Geometry: final body of the model. Coordinates: model frame, mm. Face numbers are marked on the shaded views. A direction names the side the tool comes from. Coordinates: 2 decimals unless noted, no trailing zeros. Order: outer loops, then holes, each group sorted by start corner. A loop starts at its lowest first (then second) coordinate and runs counter-clockwise, first axis right, second up. Notation, with made-up numbers: M 79,12 L 113,12 A22 ccw 113,40 Z; hole C 12,-7 d8. An arc over 180 degrees is marked long. Use CSV: the item, a comma, the result in double quotes. Start each with the question number.
1. Section query C-C on x = -75. Return the cut outline in (y, z).
2. Material intervals for line 1 (Z direction, x = 47, y = 3.25); line 2 (Y direction, x = -106.8, z = 52.5); line 3 (X direction, y = 7.75, z = 43), sorted ascending.
3. Section query A-A on x = 53. Return the cut outline in (y, z), and give its area (3 significant figures).
4. Section query B-B on z = 22.5. Return the cut outline in (x, y).
5. First-contact query: P1, Ø3, axis at x = -66.51, z = 0.57, coming from the -Y side; P2, Ø4, axis at x = 62, z = 74.5, coming from the +Y side; P3, Ø4.5, axis at x = 75, y = 5, coming from the +Z side; P4, Ø3.5, axis at x = 75, y = 5, coming from the -Z side. Flat tips, straight axial feed; report the tip coordinate or a pass-through.
6. Set-up query: the marked faces 1 and 2. Return all of +Z, -Z, +X, -X, +Y, -Y with unobstructed straight access to the full face (end or side cutting, diameter ignored); none if empty.
7. Section query D-D on z = 43. Return the cut outline in (x, y), and give its area (3 significant figures).
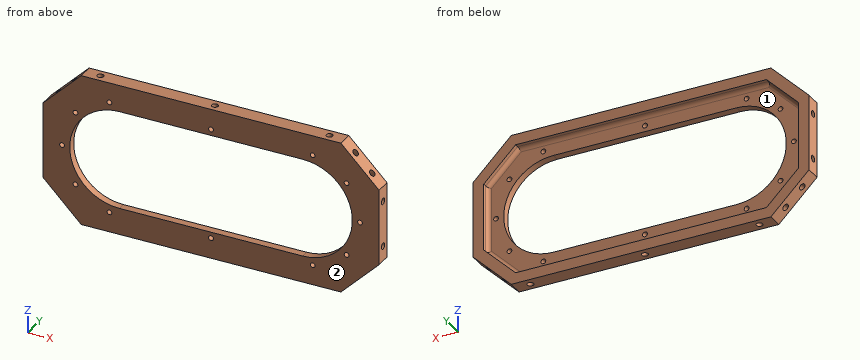
from build123d import *

# Parameters (mm, degrees)
MAIN_DEPTH                                     = 10
SKETCH3_R                                      = 1.55
ACTUATOR_SCREW_HOLE_DEPTH                      = 141.91220671
ACTUATOR_SCREW_HOLE_PATTERN_COUNT              = 3
ACTUATOR_SCREW_HOLE_PATTERN_ANGLE              = 80
ACTUATOR_SCREW_HOLE_PATTERN_THE_OTHER_WA_COUNT = 3
ACTUATOR_SCREW_HOLE_PATTERN_THE_OTHER_WA_ANGLE = 80
DISH_DEPTH                                     = 5
DISH_FILLET_R                                  = 2.5
F_4_0MM_DOWEL_HOLE1_D                          = 4.1
F_4_0MM_DOWEL_HOLE1_DEPTH                      = 5.7
F_4_0MM_DOWEL_HOLE1_ON_FACE_2_D                = 4.1
F_4_0MM_DOWEL_HOLE1_ON_FACE_2_DEPTH            = 5.7
F_4_0MM_DOWEL_HOLE1_ON_FACE_3_D                = 4.1
F_4_0MM_DOWEL_HOLE1_ON_FACE_3_DEPTH            = 5.7
F_4_0MM_DOWEL_HOLE1_ON_FACE_4_D                = 4.1
F_4_0MM_DOWEL_HOLE1_ON_FACE_4_DEPTH            = 5.7
F_4_0MM_DOWEL_HOLE1_ON_FACE_5_D                = 4.1
F_4_0MM_DOWEL_HOLE1_ON_FACE_5_DEPTH            = 5.7
F_4_0MM_DOWEL_HOLE1_ON_FACE_6_D                = 4.1
F_4_0MM_DOWEL_HOLE1_ON_FACE_6_DEPTH            = 5.7
F_4_0MM_DOWEL_HOLE1_ON_FACE_7_D                = 4.1
F_4_0MM_DOWEL_HOLE1_ON_FACE_7_DEPTH            = 5.7
F_4_0MM_DOWEL_HOLE1_ON_FACE_8_D                = 4.1
F_4_0MM_DOWEL_HOLE1_ON_FACE_8_DEPTH            = 5.7
F_4_0MM_DOWEL_HOLE1_ON_FACE_9_D                = 4.1
F_4_0MM_DOWEL_HOLE1_ON_FACE_9_DEPTH            = 5.7
F_4_0MM_DOWEL_HOLE1_ON_FACE_10_D               = 4.1
F_4_0MM_DOWEL_HOLE1_ON_FACE_10_DEPTH           = 5.7
SKETCH14_R                                     = 1.6
COVER_SRCREWHOLES_DEPTH                        = 141.91220671


with BuildPart() as part:
    # Sketch1 → Main (new body)
    with BuildSketch(Plane(origin=(0, 0, 0), x_dir=(1, 0, 0), z_dir=(0, 1, 0))):
        with BuildLine():
            Line((85, 12.5), (0, 12.5))
            Line((0, 12.5), (0, 0))
            Line((0, 0), (0, -5))
            Line((0, -5), (60, -5))
            ThreePointArc((60, -5), (92.5, -37.5), (60, -70))
            Line((60, -70), (0, -70))
            Line((0, -70), (0, -75))
            Line((0, -75), (0, -87.5))
            Line((0, -87.5), (85, -87.5))
            Line((85, -87.5), (110, -62.5))
            Line((110, -62.5), (110, -12.5))
            Line((110, -12.5), (85, 12.5))
        make_face()
    extrude(amount=MAIN_DEPTH)

    # Sketch3 → Actuator Screw Hole (cut, through all)
    with BuildSketch(Plane(origin=(0, 10, 0), x_dir=(1, 0, 0), z_dir=(0, 1, 0))):
        with Locations(Location((97.5, -37.5, 0), (0, 0, 270))):
            Circle(SKETCH3_R)
    actuator_screw_hole = extrude(amount=-ACTUATOR_SCREW_HOLE_DEPTH, mode=Mode.SUBTRACT)

    # Actuator Screw Hole Pattern: Actuator Screw Hole ×3 about axis
    actuator_screw_hole_pattern_axis = Axis((60, 0, 37.5), (0, 1, 0))
    for i in range(1, ACTUATOR_SCREW_HOLE_PATTERN_COUNT):
        add(actuator_screw_hole.rotate(actuator_screw_hole_pattern_axis, i * ACTUATOR_SCREW_HOLE_PATTERN_ANGLE / (ACTUATOR_SCREW_HOLE_PATTERN_COUNT - 1)), mode=Mode.SUBTRACT)

    # Actuator Screw Hole Pattern the other wa: Actuator Screw Hole ×3 about axis
    actuator_screw_hole_pattern_the_other_wa_axis = Axis((60, 0, 37.5), (0, -1, 0))
    for i in range(1, ACTUATOR_SCREW_HOLE_PATTERN_THE_OTHER_WA_COUNT):
        add(actuator_screw_hole.rotate(actuator_screw_hole_pattern_the_other_wa_axis, i * ACTUATOR_SCREW_HOLE_PATTERN_THE_OTHER_WA_ANGLE / (ACTUATOR_SCREW_HOLE_PATTERN_THE_OTHER_WA_COUNT - 1)), mode=Mode.SUBTRACT)

    # Mirror1: part across plane


with BuildPart() as part_1:
    add(part.part)
    add(part.part.mirror(Plane(origin=(0, 0, 0), x_dir=(0, 0, 1), z_dir=(1, 0, 0))))

    # Sketch8 → Dish (cut)
    with BuildSketch(Plane(origin=(0, 10, 0), x_dir=(1, 0, 0), z_dir=(0, 1, 0))):
        Polygon((82.100505063, 5.5), (-82.100505063, 5.5), (-103, -15.399494937), (-103, -59.600505063), (-82.100505063, -80.5), (82.100505063, -80.5), (103, -59.600505063), (103, -15.399494937), align=None)
    extrude(amount=-DISH_DEPTH, mode=Mode.SUBTRACT)

    # Dish fillet
    dish_fillet_edges = [part_1.edges().sort_by_distance(p)[0] for p in [
        (92.550252532, 5, 4.949747468),
        (103, 5, 37.5),
        (92.550252532, 5, 70.050252532),
        (0, 5, 80.5),
        (-92.550252532, 5, 70.050252532),
        (-103, 5, 37.5),
        (-92.550252532, 5, 4.949747468),
        (0, 5, -5.5),
    ]]
    fillet(dish_fillet_edges, radius=DISH_FILLET_R)

    # Ø4.0mm Dowel Hole1
    with Locations(Plane(origin=(75, 5, -12.5), x_dir=(-1, 0, 0), z_dir=(0, 0, -1))):
        with Locations((0, 0), (75, 0), (150, 0)):
            Hole(F_4_0MM_DOWEL_HOLE1_D / 2, depth=F_4_0MM_DOWEL_HOLE1_DEPTH)

    # Ø4.0mm Dowel Hole1 on face 2
    with Locations(Plane(origin=(-92.071067812, 5, -5.428932188), x_dir=(-0.707106781187, 0, 0.707106781187), z_dir=(-0.707106781187, 0, -0.707106781187))):
        with Locations((0, 0), (15.355339059, 0)):
            Hole(F_4_0MM_DOWEL_HOLE1_ON_FACE_2_D / 2, depth=F_4_0MM_DOWEL_HOLE1_ON_FACE_2_DEPTH)

    # Ø4.0mm Dowel Hole1 on face 3
    with Locations(Plane(origin=(-110, 5, 22.5), x_dir=(0, 0, -1), z_dir=(-1, 0, 0))):
        with Locations((0, 0), (-30, 0)):
            Hole(F_4_0MM_DOWEL_HOLE1_ON_FACE_3_D / 2, depth=F_4_0MM_DOWEL_HOLE1_ON_FACE_3_DEPTH)

    # Ø4.0mm Dowel Hole1 on face 4
    with Locations(Plane(origin=(-102.928932188, 5, 69.571067812), x_dir=(0.707106781187, 0, 0.707106781187), z_dir=(-0.707106781187, 0, 0.707106781187))):
        with Locations((0, 0)):
            Hole(F_4_0MM_DOWEL_HOLE1_ON_FACE_4_D / 2, depth=F_4_0MM_DOWEL_HOLE1_ON_FACE_4_DEPTH)

    # Ø4.0mm Dowel Hole1 on face 5
    with Locations(Plane(origin=(-92.071067812, 5, 80.428932188), x_dir=(0.707106781187, 0, 0.707106781187), z_dir=(-0.707106781187, 0, 0.707106781187))):
        with Locations((0, 0)):
            Hole(F_4_0MM_DOWEL_HOLE1_ON_FACE_5_D / 2, depth=F_4_0MM_DOWEL_HOLE1_ON_FACE_5_DEPTH)

    # Ø4.0mm Dowel Hole1 on face 6
    with Locations(Plane(origin=(-75, 5, 87.5), x_dir=(1, 0, 0), z_dir=(0, 0, 1))):
        with Locations((0, 0), (75, 0), (150, 0)):
            Hole(F_4_0MM_DOWEL_HOLE1_ON_FACE_6_D / 2, depth=F_4_0MM_DOWEL_HOLE1_ON_FACE_6_DEPTH)

    # Ø4.0mm Dowel Hole1 on face 7
    with Locations(Plane(origin=(92.071067812, 5, 80.428932188), x_dir=(0.707106781187, 0, -0.707106781187), z_dir=(0.707106781187, 0, 0.707106781187))):
        with Locations((0, 0)):
            Hole(F_4_0MM_DOWEL_HOLE1_ON_FACE_7_D / 2, depth=F_4_0MM_DOWEL_HOLE1_ON_FACE_7_DEPTH)

    # Ø4.0mm Dowel Hole1 on face 8
    with Locations(Plane(origin=(102.928932188, 5, 69.571067812), x_dir=(0.707106781187, 0, -0.707106781187), z_dir=(0.707106781187, 0, 0.707106781187))):
        with Locations((0, 0)):
            Hole(F_4_0MM_DOWEL_HOLE1_ON_FACE_8_D / 2, depth=F_4_0MM_DOWEL_HOLE1_ON_FACE_8_DEPTH)

    # Ø4.0mm Dowel Hole1 on face 9
    with Locations(Plane(origin=(110, 5, 52.5), x_dir=(0, 0, 1), z_dir=(1, 0, 0))):
        with Locations((0, 0), (-30, 0)):
            Hole(F_4_0MM_DOWEL_HOLE1_ON_FACE_9_D / 2, depth=F_4_0MM_DOWEL_HOLE1_ON_FACE_9_DEPTH)

    # Ø4.0mm Dowel Hole1 on face 10
    with Locations(Plane(origin=(102.928932188, 5, 5.428932188), x_dir=(-0.707106781187, 0, -0.707106781187), z_dir=(0.707106781187, 0, -0.707106781187))):
        with Locations((0, 0), (15.355339059, 0)):
            Hole(F_4_0MM_DOWEL_HOLE1_ON_FACE_10_D / 2, depth=F_4_0MM_DOWEL_HOLE1_ON_FACE_10_DEPTH)

    # Sketch14 → Cover srcrewholes (cut, through all)
    with BuildSketch(Plane.XZ):
        with Locations(Location((0, 1, 0), (0, 0, 270))):
            Circle(SKETCH14_R)
        with Locations(Location((0, 74, 0), (0, 0, 270))):
            Circle(SKETCH14_R)
    extrude(amount=-COVER_SRCREWHOLES_DEPTH, mode=Mode.SUBTRACT)


solid = part_1.part
Results list:
1,outline,"M 0,-12.5 L 2.95,-12.5 L 2.95,-6.8 L 7.05,-6.8 L 7.05,-12.5 L 10,-12.5 L 10,-5.5 L 7.5,-5.5 A2.5 cw 5,-3 L 5,8.67 L 0,8.67 Z; M 0,66.33 L 5,66.33 L 5,78 A2.5 cw 7.5,80.5 L 10,80.5 L 10,87.5 L 7.05,87.5 L 7.05,81.8 L 2.95,81.8 L 2.95,87.5 L 0,87.5 Z"
2,line 1,"z = -12.5 to 5, 70 to 87.5"
2,line 2,"y = 0 to 2.95, 7.05 to 10"
2,line 3,"x = -110 to -103, 103 to 110"
3,outline,"M 0,-12.5 L 10,-12.5 L 10,-5.5 L 7.5,-5.5 A2.5 cw 5,-3 L 5,5 L 0,5 Z; M 0,70 L 5,70 L 5,78 A2.5 cw 7.5,80.5 L 10,80.5 L 10,87.5 L 0,87.5 Z"
3,area,"248 mm²"
4,outline,"M -110,0 L -88.83,0 L -88.83,5 L -100.5,5 A2.5 cw -103,7.5 L -103,10 L -110,10 L -110,7.05 L -104.3,7.05 L -104.3,2.95 L -110,2.95 Z; M 88.83,0 L 110,0 L 110,2.95 L 104.3,2.95 L 104.3,7.05 L 110,7.05 L 110,10 L 103,10 L 103,7.5 A2.5 cw 100.5,5 L 88.83,5 Z"
5,P1,"passes through"
5,P2,"stops at y = 5"
5,P3,"stops at z = 87.5"
5,P4,"stops at z = -6.8"
6,face 1,"+Y"
6,face 2,"+Z, -Z, +X, -X, -Y"
7,outline,"M -110,0 L -92.03,0 L -92.03,5 L -100.5,5 A2.5 cw -103,7.5 L -103,10 L -110,10 Z; M 92.03,0 L 110,0 L 110,10 L 103,10 L 103,7.5 A2.5 cw 100.5,5 L 92.03,5 Z"
7,area,"252 mm²"
